Check sheet for the modelled part. Datum: model origin and axes. Units: mm. A direction names the side the tool comes from. Coordinates: 2 decimals unless noted, no trailing zeros. Loops run counter-clockwise (first coordinate to the right, second up) from the corner with the lowest first, then second, coordinate; pieces in that order, holes last. Notation, with made-up numbers: (-28.5, 30) -> (29.5, 30) arc R21 ccw to (29.5, 51) -> close; hole circle Ø9 at (2.5, 22.25). An arc over 180 degrees is marked (long way). Use CSV: the item, a comma, the result in double quotes. Start each with the question number.
1. Gauge pin test, flat ends, axial feed: pin 1 (1.9 mm diameter, centred on x = -17.5, y = 31, fed in from +Z); pin 2 (2.5 mm diameter, centred on x = -25, y = 37, fed in from +Z). Record the tip position at first contact, or that the pin passes through.
2. Sectioned sample at D-D, the plane y = 8. Record the cut outline in (x, z).
3. Set-up check for faces 1 (the face through (-39.56, 24, 8)), 2 (the face through (-17, 36, 11.673)), 3 (the face through (-24, 22, 8)), 4 (the face through (-28.01, 36, 14)): record each of +Z, -Z, +X, -X, +Y, -Y from which the full face is reachable in a straight line by a thin tool's end or side.
4. Sectioned sample at C-C, the plane y = 41. Record the cut outline in (x, z), and give its area (3 significant figures).
5. Sectioned sample at B-B, the plane x = -16.5. Record the cut outline in (y, z).
6. Thickness scan on L1, parallel to X at y = 46, z = 10.5; L2, parallel to X at y = 28.5, z = 14.25; L3, parallel to Z at x = -27.5, y = 47. Record the ranges inside material, lowest first.
7. Sectioned sample at A-A, the plane z = 15.5. Record the cut outline in (x, y), and give its area (3 significant figures).
```python
from build123d import *

# Parameters (mm, degrees)
ESQUISSE1_W                  = 30.8
ESQUISSE1_H                  = 24.15
BOSS_EXTRU_1_DEPTH           = 49
ESQUISSE3_R                  = 2.75
ENL_V_MAT_EXTRU_3_DEPTH      = 22
ENL_V_MAT_EXTRU_4_DEPTH      = 67.174451426
ENL_V_MAT_EXTRU_4_DEPTH_BACK = 25


with BuildPart() as part:
    # Esquisse1 → Boss.-Extru.1 (new body)
    with BuildSketch(Plane(origin=(0, 0, 0), x_dir=(1, 0, 0), z_dir=(0, 1, 0))):
        with Locations((-24.160479042, -8.248053892)):
            Rectangle(ESQUISSE1_W, ESQUISSE1_H)
    extrude(amount=BOSS_EXTRU_1_DEPTH)

    # Esquisse3 → Enlèv. mat.-Extru.3 (cut)
    with BuildSketch(Plane(origin=(0, 0, 0), x_dir=(-1, 0, 0), z_dir=(0, -1, 0))):
        with Locations(Location((24.160479042, -8.323053892, 0), (0, 0, 90))):
            Circle(ESQUISSE3_R)
    extrude(amount=-ENL_V_MAT_EXTRU_3_DEPTH, mode=Mode.SUBTRACT)

    # Esquisse2 → Enlèv. mat.-Extru.4 (cut, two sides: drawn at the far end of the back side and taken through both)
    with BuildSketch(Plane(origin=(0, 49, 0), x_dir=(1, 0, 0), z_dir=(0, 1, 0)).offset(-ENL_V_MAT_EXTRU_4_DEPTH_BACK)):
        Polygon((-34.260479042, -100.564708201), (-34.260479042, -20.323053892), (-34.260479042, -16.473053892), (-28.010479042, -16.473053892), (-28.010479042, -11.673053892), (-34.260479042, -11.673053892), (-34.260479042, -3.973053892), (-26.560479042, -3.973053892), (-26.560479042, -10.223053892), (-21.760479042, -10.223053892), (-21.760479042, -3.973053892), (-14.060479042, -3.973053892), (-14.060479042, -11.673053892), (-20.310479042, -11.673053892), (-20.310479042, -16.473053892), (-14.060479042, -16.473053892), (-14.060479042, -20.323053892), (-14.060479042, -100.564708201), (-14.060479042, -261.048016818), (-34.260479042, -261.048016818), align=None)
    extrude(amount=ENL_V_MAT_EXTRU_4_DEPTH + ENL_V_MAT_EXTRU_4_DEPTH_BACK, mode=Mode.SUBTRACT)


solid = part.part
```
Completed:
1,pin 1,"z = 16.47"
1,pin 2,"z = 10.22"
2,outline,"(-39.56, -3.83) -> (-8.76, -3.83) -> (-8.76, 20.32) -> (-39.56, 20.32) -> close; hole circle Ø5.5 at (-24.16, 8.32)"
3,face 1,"+Z, -Z, -X, +Y, -Y"
3,face 2,"+Y"
3,face 3,"-Y"
3,face 4,"+Z, +Y"
4,outline,"(-39.56, -3.83) -> (-8.76, -3.83) -> (-8.76, 20.32) -> (-14.06, 20.32) -> (-14.06, 16.47) -> (-20.31, 16.47) -> (-20.31, 11.67) -> (-14.06, 11.67) -> (-14.06, 3.97) -> (-21.76, 3.97) -> (-21.76, 10.22) -> (-26.56, 10.22) -> (-26.56, 3.97) -> (-34.26, 3.97) -> (-34.26, 11.67) -> (-28.01, 11.67) -> (-28.01, 16.47) -> (-34.26, 16.47) -> (-34.26, 20.32) -> (-39.56, 20.32) -> close"
4,area,"504 mm²"
5,outline,"(0, -3.83) -> (49, -3.83) -> (49, 3.97) -> (24, 3.97) -> (24, 11.67) -> (49, 11.67) -> (49, 16.47) -> (24, 16.47) -> (24, 20.32) -> (0, 20.32) -> close"
6,L1,"-39.56 to -34.26, -14.06 to -8.76"
6,L2,"-39.56 to -28.01, -20.31 to -8.76"
6,L3,"-3.83 to 3.97"
7,outline,"(-39.56, 0) -> (-8.76, 0) -> (-8.76, 49) -> (-20.31, 49) -> (-20.31, 24) -> (-28.01, 24) -> (-28.01, 49) -> (-39.56, 49) -> close"
7,area,"1,320 mm²"
